The figure shows three views and two pictorial views of one solid part (mm, origin at its lowest corner). Answer the questions. Coordinates: 2 decimals unless noted, no trailing zeros. Order: outer loops, then holes, each group sorted by start corner. A loop starts at its lowest first (then second) coordinate and runs counter-clockwise, first axis right, second up. Notation, with made-up numbers: (-1, -26.75) -> (32, -26.75) arc R21 cw to (32, 2.25) -> close; hole circle Ø10 at (81, 53.5). An arc over 180 degrees is marked (long way). Return JSON: item names as keys, results as strings.
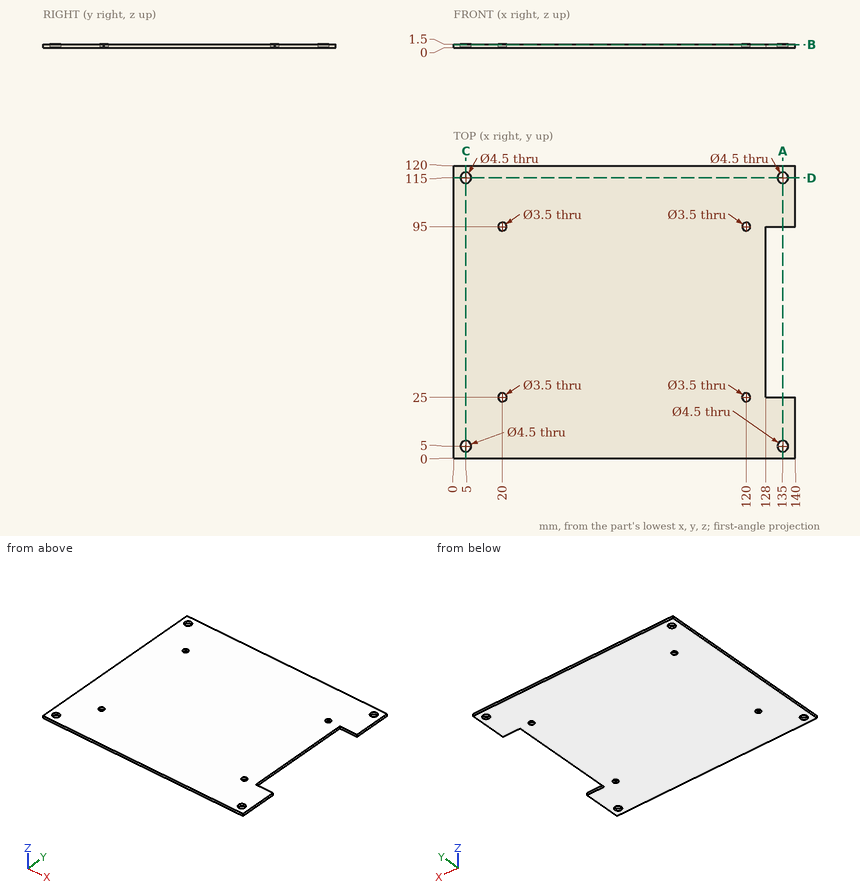
1. This flat-tipped pin is pushed along its axis until it touches: pin 1 Ø0.8 at (y, z) = (76, 1) entering from +X. Where does it stop, or does it pass through?
Answer block:
{"pin 1": "stops at x = 128"}
2. The part is cut by section A-A on x = 135. Give the vertices of the cut face in (y, z).
Answer block:
{"outline": "(0, 0) -> (2.75, 0) -> (2.75, 1.5) -> (0, 1.5) -> close; (7.25, 0) -> (25, 0) -> (25, 1.5) -> (7.25, 1.5) -> close; (95, 0) -> (112.75, 0) -> (112.75, 1.5) -> (95, 1.5) -> close; (117.25, 0) -> (120, 0) -> (120, 1.5) -> (117.25, 1.5) -> close"}
3. Consider line 1 (Y direction, x = 135, z = 0.65); line 2 (Y direction, x = 120, z = 1.2); line 3 (X direction, y = 25.5, z = 1.1). Determine where each line is inside the solid, lowest interval first. Write a range as from..to.
Answer block:
{"line 1": "y = 0..2.75, 7.25..25, 95..112.75, 117.25..120", "line 2": "y = 0..23.25, 26.75..93.25, 96.75..120", "line 3": "x = 0..18.32, 21.68..118.32, 121.68..128"}
4. The part is cut by section B-B on z = 1.2. Give the number of separate pieces and of enclosed holes in the cut face, and give its area (3 significant figures).
Answer block:
{"separate pieces": "1", "enclosed holes": "8", "area": "15,900 mm2"}
5. The part is cut by section C-C on x = 5. Give the vertices of the cut face in (y, z), and give its area (4 significant figures).
Answer block:
{"outline": "(0, 0) -> (2.75, 0) -> (2.75, 1.5) -> (0, 1.5) -> close; (7.25, 0) -> (112.75, 0) -> (112.75, 1.5) -> (7.25, 1.5) -> close; (117.25, 0) -> (120, 0) -> (120, 1.5) -> (117.25, 1.5) -> close", "area": "166.5 mm2"}
6. The part is cut by section D-D on y = 115. Give the vertices of the cut face in (x, z), and give its area (4 significant figures).
Answer block:
{"outline": "(0, 0) -> (2.75, 0) -> (2.75, 1.5) -> (0, 1.5) -> close; (7.25, 0) -> (132.75, 0) -> (132.75, 1.5) -> (7.25, 1.5) -> close; (137.25, 0) -> (140, 0) -> (140, 1.5) -> (137.25, 1.5) -> close", "area": "196.5 mm2"}
